For this review, use the dimensioned drawing (mm, ordinates from the lowest corner) and the shaded views. A direction names the side the tool comes from. Coordinates: 2 decimals unless noted, no trailing zeros. Write each loop counter-clockwise with the first axis right and the second up, starting at its lowest first coordinate (ties: lowest second). Pieces come first, ordered by that corner, then holes. Notation, with made-up numbers: (71, 24.5) - (112, 24.5) arc R19 ccw to (112, 60.5) - close; hole circle Ø2 at (-24, 49.5). An arc over 180 degrees is marked (long way). Answer as a JSON object with one key per item and string values.
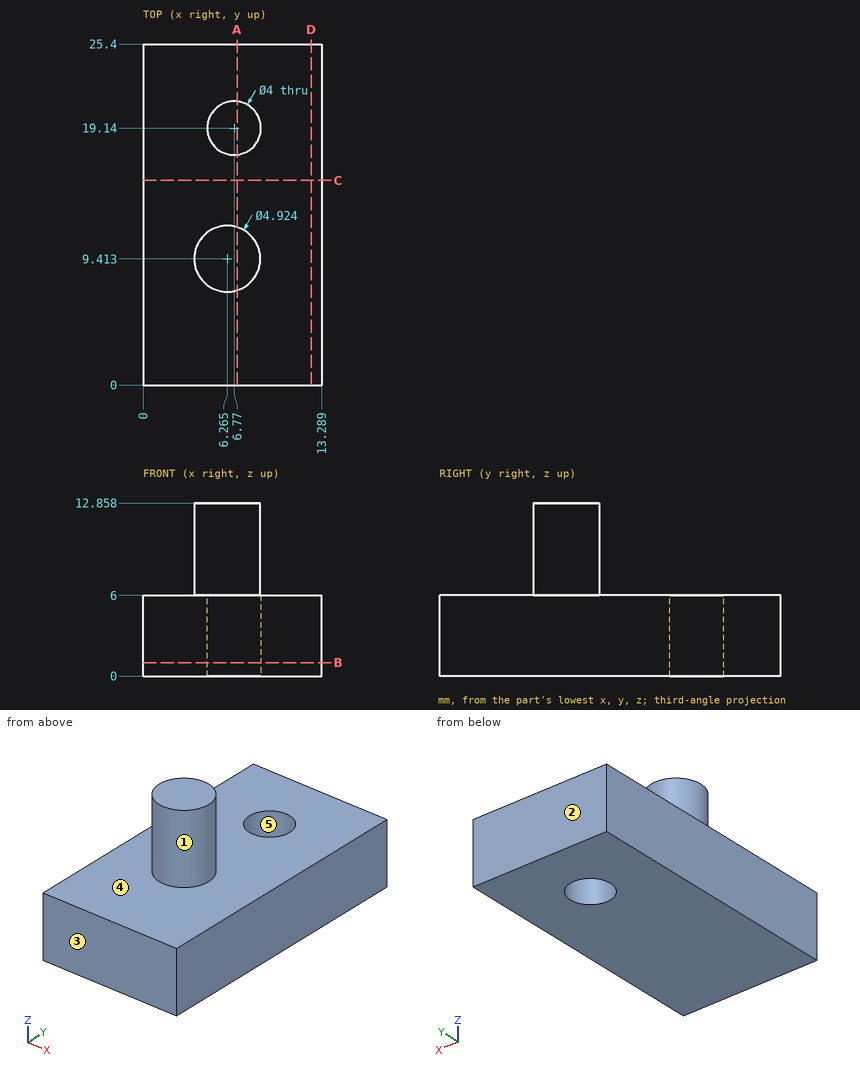
(1) To check wall thickness, follow line 1 (Z direction, x = 6.5, y = 2); line 2 (Y direction, x = 5.25, z = 1); line 3 (X direction, y = 18, z = 3.25) (1 decimal). State the ranges of each line that lie inside material, in increasing order. Write a range as from..to.
Solved:
{"line 1": "z = 0..6", "line 2": "y = 0..17.84, 20.44..25.4", "line 3": "x = 0..5.1, 8.4..13.3"}
(2) Tool access review of the marked faces 1 and 2: name each direction out of +Z, -Z, +X, -X, +Y, -Y from which nothing blocks a thin tool from reaching the whole face with its end or side.
Solved:
{"face 1": "+Z", "face 2": "+Z, -Z, +X, -X, +Y"}
(3) Take a section at C-C, the plane y = 15.25. Write out the cut boundary in (x, z).
Solved:
{"outline": "(0, 0) - (13.29, 0) - (13.29, 6) - (0, 6) - close"}
(4) Take a section at A-A, the plane x = 7. Write out the cut boundary in (y, z).
Solved:
{"outline": "(0, 0) - (17.15, 0) - (17.15, 6) - (11.76, 6) - (11.76, 12.86) - (7.06, 12.86) - (7.06, 6) - (0, 6) - close; (21.13, 0) - (25.4, 0) - (25.4, 6) - (21.13, 6) - close"}
(5) Take a section at B-B, the plane z = 1. Write out the cut boundary in (x, y).
Solved:
{"outline": "(0, 0) - (13.29, 0) - (13.29, 25.4) - (0, 25.4) - close; hole circle Ø4 at (6.77, 19.14)"}
(6) Take a section at D-D, the plane x = 12.5. Write out the cut boundary in (y, z).
Solved:
{"outline": "(0, 0) - (25.4, 0) - (25.4, 6) - (0, 6) - close"}
(7) The part is to be moulded in two halves that separate along Y. For the marked faces 3, 4 and 5, say which applies: pulls with the +Y half, pulls with the -Y half, needs draft (parallel to the pull), parting line crosses it, or undercut.
Solved:
{"face 3": "pulls with the -Y half", "face 4": "needs draft", "face 5": "undercut"}
